from build123d import *

# Parameters (mm, degrees)
SKETCH1_R           = 1.75
BOSS_EXTRUDE1_DEPTH = 19.304
CUT_EXTRUDE1_START  = -19.304
CUT_EXTRUDE1_DEPTH  = 17.78


with BuildPart() as part:
    # Sketch1 → Boss-Extrude1 (new body)
    with BuildSketch(Plane(origin=(0, 0, 0), x_dir=(1, 0, 0), z_dir=(0, 1, 0))):
        with BuildLine():
            Line((-7.239, -11.948128682), (-7.239, -15.65830815))
            Line((-7.239, -15.65830815), (7.239, -15.65830815))
            Line((7.239, -15.65830815), (7.239, -11.948128682))
            ThreePointArc((7.239, -11.948128682), (11.19086866, -8.362138401), (13.509839525, -3.556))
            Line((13.509839525, -3.556), (18.139005902, -3.556))
            ThreePointArc((18.139005902, -3.556), (19.935057126, -2.812051224), (20.679005902, -1.016))
            Line((20.679005902, -1.016), (20.679005902, 0.904))
            ThreePointArc((20.679005902, 0.904), (19.935057126, 2.700051224), (18.139005902, 3.444))
            Line((18.139005902, 3.444), (13.538824321, 3.444))
            ThreePointArc((13.538824321, 3.444), (0, 13.97), (-13.538824321, 3.444))
            Line((-13.538824321, 3.444), (-18.305445148, 3.444))
            ThreePointArc((-18.305445148, 3.444), (-20.101496373, 2.700051224), (-20.845445148, 0.904))
            Line((-20.845445148, 0.904), (-20.845445148, -1.016))
            ThreePointArc((-20.845445148, -1.016), (-20.101496373, -2.812051224), (-18.305445148, -3.556))
            Line((-18.305445148, -3.556), (-13.509839525, -3.556))
            ThreePointArc((-13.509839525, -3.556), (-11.19086866, -8.362138401), (-7.239, -11.948128682))
        make_face()
        with Locations((17.499965, 0)):
            Circle(SKETCH1_R, mode=Mode.SUBTRACT)
        with Locations((-17.499965, 0)):
            Circle(SKETCH1_R, mode=Mode.SUBTRACT)
    extrude(amount=BOSS_EXTRUDE1_DEPTH)

    # Sketch2 → Cut-Extrude1 (cut)
    with BuildSketch(Plane(origin=(0, 19.304, 0), x_dir=(1, 0, 0), z_dir=(0, 1, 0)).offset(CUT_EXTRUDE1_START)):
        with BuildLine():
            Line((-13.538824321, 3.444), (-18.305445148, 3.444))
            Line((-18.305445148, 3.444), (-22.379136798, 3.444))
            Line((-22.379136798, 3.444), (-22.379136798, -3.598718101))
            Line((-22.379136798, -3.598718101), (-18.305445148, -3.556))
            Line((-18.305445148, -3.556), (-13.509839525, -3.556))
            ThreePointArc((-13.509839525, -3.556), (-13.969880242, -0.057844875), (-13.538824321, 3.444))
        make_face()
        with BuildLine():
            Line((18.305445148, -3.556), (13.509839525, -3.556))
            ThreePointArc((13.509839525, -3.556), (13.969880242, -0.057844875), (13.538824321, 3.444))
            Line((13.538824321, 3.444), (18.305445148, 3.444))
            ThreePointArc((18.305445148, 3.444), (20.101496373, 2.700051224), (20.845445148, 0.904))
            Line((20.845445148, 0.904), (20.777862254, -1.598025477))
            ThreePointArc((20.777862254, -1.598025477), (19.998954522, -3.154465794), (18.305445148, -3.556))
        make_face()
    extrude(amount=CUT_EXTRUDE1_DEPTH, mode=Mode.SUBTRACT)


solid = part.part
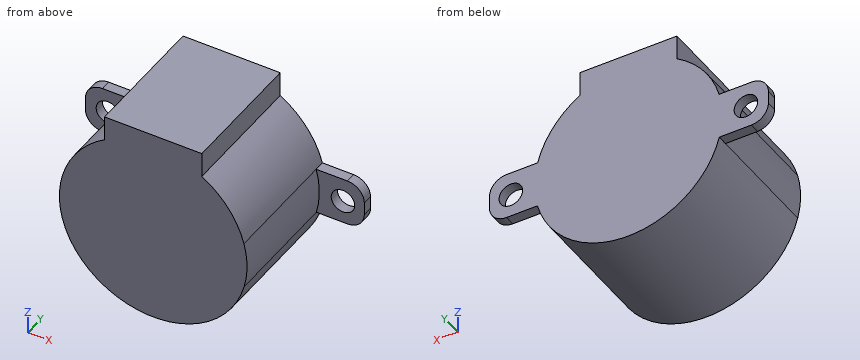
Design review of the part built by this model. Coordinates are the model's own, in mm. Coordinates: 2 decimals unless noted, no trailing zeros. Order: outer loops, then holes, each group sorted by start corner. A loop starts at its lowest first (then second) coordinate and runs counter-clockwise, first axis right, second up.
Item 1: Take a section at A-A, the plane z = 0. Write out the cut boundary in (x, y), then the cut area to 3 significant figures.
Item 2: Take a section at D-D, the plane x = -13. Write out the cut boundary in (y, z).
Item 3: For pin 1 Ø1.9 at (y, z) = (7.5, 13) entering from -X; pin 2 Ø0.5 at (x, y) = (-15, 18.5) entering from +Z; pin 3 Ø3.5 at (x, z) = (15.5, 1) entering from -Y; pin 4 Ø1.2 at (x, y) = (17, 18) entering from -Z, all flat-tipped, find the tip position at first contact; note any pin that passes through.
Item 4: For line 1 (X direction, y = 18.9, z = 0); line 2 (X direction, y = 18.75, z = -0.25); line 3 (X direction, y = 8.5, z = 12), list the stretches that pass through material, from the lowest coordinate up.
Item 5: Take a section at C-C, the plane z = 13.5. Write out the cut boundary in (x, y).
Item 6: Take a section at B-B, the plane y = 15.5. Write out the cut boundary in (x, z).
The answers:
1. outline: (-20.85, 17.78) - (-19.25, 17.78) - (-19.25, 19.3) - (-20.85, 19.3) - close; (-15.75, 17.78) - (-13.97, 17.78) - (-13.97, 0) - (13.97, 0) - (13.97, 17.78) - (15.75, 17.78) - (15.75, 19.3) - (-15.75, 19.3) - close; (19.25, 17.78) - (20.68, 17.78) - (20.68, 19.3) - (19.25, 19.3) - close
1. area: 549 mm2
2. outline: (0, -5.11) - (19.3, -5.11) - (19.3, 5.11) - (0, 5.11) - close
3. pin 1: stops at x = -7.24
3. pin 2: stops at z = 3.56
3. pin 3: stops at y = 0
3. pin 4: stops at z = -3.44
4. line 1: x = -20.85 to -19.25, -15.75 to 15.75, 19.25 to 20.68
4. line 2: x = -20.85 to -19.23, -15.77 to 15.77, 19.23 to 20.68
4. line 3: x = -7.24 to 7.24
5. outline: (-7.24, 0) - (7.24, 0) - (7.24, 19.3) - (-7.24, 19.3) - close
6. outline: (-7.24, 11.95) arc R13.97 ccw (long way) to (7.24, 11.95) - (7.24, 15.66) - (-7.24, 15.66) - close
